Geometry: final body of the model. Coordinates: model frame, mm. A direction names the side the tool comes from. Round coordinates to 2 decimals unless told otherwise and drop trailing zeros. Loops run counter-clockwise (first coordinate to the right, second up) from the corner with the lowest first, then second, coordinate; pieces in that order, holes last. Notation, with made-up numbers: (84, 27.25) -> (110, 27.25) arc R10 cw to (110, 31.25) -> close; hole circle Ø2 at (12, 64). An arc over 180 degrees is marked (long way). Answer in a Markdown table with one row per item.
Autodesk Fusion 360 part; units mm, degrees
sketch "Sketch1" plane through (0, 0, 0) normal (0, 0, 1) x (1, 0, 0)
  line L0 (14.71, 7.35) -> (-14.71, 7.35)
  line L1 (-14.71, 7.35) -> (-14.71, -7.35)
  line L2 (-14.71, -7.35) -> (14.71, -7.35)
  line L3 (14.71, -7.35) -> (14.71, 7.35)
  line L4 (14.71, 7.35) -> (-14.71, -7.35) construction
  line L5 (-14.71, 7.35) -> (14.71, -7.35) construction
  line L6 (-17.7, 7.35) -> (-17.7, 14.7)
  line L7 (-17.7, 14.7) -> (-14.71, 14.7)
  line L8 (-17.7, 14.7) -> (17.7, 14.7)
  line L9 (17.7, 14.7) -> (17.7, -18.8)
  line L10 (17.7, -18.8) -> (-17.7, -18.8)
  line L11 (-17.7, -18.8) -> (-17.7, 14.7)
  line L12 (-17.7, 14.7) -> (6.5694, 14.7)
  line L13 (6.5694, 9.45) -> (-14.71, 9.45)
  line L14 (-17.7, 9.45) -> (-17.7, 14.7)
  line L15 (17.7, 9.45) -> (-17.7, 9.45)
  line L16 (-17.7, 9.45) -> (-17.7, -13.55)
  line L17 (-17.7, -13.55) -> (17.7, -13.55)
  line L18 (17.7, -13.55) -> (17.7, 9.45)
  line L19 (-17.7, 14.7) -> (-15.2, 14.7)
  line L20 (-15.2, 14.7) -> (-15.2, 12.2)
  line L21 (-15.2, 12.2) -> (-17.7, 12.2)
  line L22 (-17.7, 12.2) -> (-17.7, 14.7)
  circle A0 centre (-15.2, 12.2) radius 1.5
  circle A1 centre (15.2, 12.2) radius 1.5
  circle A2 centre (-15.2, -16.3) radius 1.5
  circle A3 centre (15.2, -16.3) radius 1.5
  line L23 (-17.7, -18.8) -> (-7, -18.8)
  line L24 (-7, -18.8) -> (-7, -17.6734)
  line L25 (-7, -17.6734) -> (-17.7, -17.6734)
  line L26 (-17.7, -17.6734) -> (-17.7, -18.8)
  line L27 (-7, -18.8) -> (7, -18.8)
  line L28 (7, -18.8) -> (7, -15.8)
  line L29 (7, -15.8) -> (-7, -15.8)
  line L30 (-7, -15.8) -> (-7, -18.8)
  line L31 (-17.7, 14.7) -> (-3.81, 14.7)
  line L32 (-3.81, 14.7) -> (-3.81, 12.7)
  line L33 (-3.81, 12.7) -> (-17.7, 12.7)
  line L34 (-17.7, 12.7) -> (-17.7, 14.7)
  circle A4 centre (-3.81, 12.7) radius 1
  circle A5 centre (-3.81, 12.7) radius 1
  circle A6 centre (-3.81, 12.7) radius 1
  circle A7 centre (-1.27, 12.7) radius 1
  circle A8 centre (1.27, 12.7) radius 1
  circle A9 centre (3.81, 12.7) radius 1
  circle A10 centre (-3.81, 12.7) radius 0.5
  circle A11 centre (-1.27, 12.7) radius 0.5
  circle A12 centre (1.27, 12.7) radius 0.5
  circle A13 centre (3.81, 12.7) radius 0.5
  line L35 (-2.81, 13.7) -> (-4.81, 13.7)
  line L36 (-4.81, 13.7) -> (-4.81, 11.7)
  line L37 (-4.81, 11.7) -> (-2.81, 11.7)
  line L38 (-2.81, 11.7) -> (-2.81, 13.7)
  line L39 (-2.81, 13.7) -> (-4.81, 11.7) construction
  line L40 (-4.81, 13.7) -> (-2.81, 11.7) construction
  line L41 (-0.27, 13.7) -> (-2.27, 13.7)
  line L42 (-2.27, 13.7) -> (-2.27, 11.7)
  line L43 (-2.27, 11.7) -> (-0.27, 11.7)
  line L44 (-0.27, 11.7) -> (-0.27, 13.7)
  line L45 (-0.27, 13.7) -> (-2.27, 11.7) construction
  line L46 (-2.27, 13.7) -> (-0.27, 11.7) construction
  line L47 (2.27, 13.7) -> (0.27, 13.7)
  line L48 (0.27, 13.7) -> (0.27, 11.7)
  line L49 (0.27, 11.7) -> (2.27, 11.7)
  line L50 (2.27, 11.7) -> (2.27, 13.7)
  line L51 (2.27, 13.7) -> (0.27, 11.7) construction
  line L52 (0.27, 13.7) -> (2.27, 11.7) construction
  line L53 (4.81, 13.7) -> (2.81, 13.7)
  line L54 (2.81, 13.7) -> (2.81, 11.7)
  line L55 (2.81, 11.7) -> (4.81, 11.7)
  line L56 (4.81, 11.7) -> (4.81, 13.7)
  line L57 (4.81, 13.7) -> (2.81, 11.7) construction
  line L58 (2.81, 13.7) -> (4.81, 11.7) construction
  point P0 (-3.81, 12.7)
  point P1 (-1.27, 12.7)
  point P2 (1.27, 12.7)
  point P3 (3.81, 12.7)
  dimension "d1" = 29.42
  dimension "d2" = 14.7
  dimension "d3" = 2.99
  dimension "d5" = 35.4
  dimension "d6" = 33.5
  dimension "d7" = 5.25
  dimension "d8" = 23
  dimension "d9" = 2.5
  dimension "d10" = 2.5
  dimension "d11" = 3
  dimension "d12" = 3
  dimension "d13" = 3
  dimension "d14" = 3
  dimension "d19" = 10.7
  dimension "d20" = 14
  dimension "d21" = 3
  dimension "d24" = 13.89
  dimension "d25" = 2
  dimension "d26" = 2
  dimension "d27" = 2
  dimension "d28" = 2
  dimension "d29" = 2
  dimension "d30" = 2
  dimension "d31" = 2
  dimension "d34" = 1
  dimension "d35" = 1
  dimension "d36" = 1
  dimension "d37" = 1
  dimension "d42" = 2
  dimension "d43" = 2
  dimension "d44" = 2
  dimension "d45" = 2
  dimension "d46" = 2
  dimension "d47" = 2
  dimension "d48" = 2
  dimension "d49" = 2
extrude "Extrude1" add sketch "Sketch1" along normal blind 1.2 contours L0 L1 L2 L3 | L6 L9 L11 L13 L15 L16 L17 L18 | L6 L8 L9 L11 L12 L13 L14 L15 L21 A0 L32 L33 L35 L36 L37 L38 | L9 L10 L11 L17 A2 L25 L28 L29 L30 | L6 L11 L14 L21 L22 A0 L33 | L10 L11 A2 L23 L24 L25 L26 L30 | L6 L7 L8 L11 L12 L14 L19 L20 L22 A0 L31 L33 L34 | L10 L24 L27 L28 L29 L30 | L7 L8 L12 L20 A0 L31 L32 L33 L35 L36 | L32 L33 A4 A5 A6 A10 | A4 A5 A6 L35 L36 | L32 L33 A4 A5 A6 A10 | A4 A5 A6 L36 L37 | L32 L33 A10 | L32 L33 A10 | A4 A5 A6 L35 L38 | A4 A5 A6 L37 L38 | A7 | A7 L43 L44 | A7 L41 L44 | A7 L41 L42 | A7 L42 L43 | A8 | A8 L49 L50 | A8 L47 L50 | A8 L47 L48 | A8 L48 L49 | A9 | A9 L55 L56 | A9 L53 L56 | A9 L53 L54 | A9 L54 L55 | A11 | A12 | A13 makes body 1
extrude "Extrude2" add sketch "Sketch1" along normal blind 2.7 contours L0 L1 L2 L3 | L6 L9 L11 L13 L15 L16 L17 L18 bodies 1
extrude "Extrude3" cut sketch "Sketch1" along normal blind 1.2 contours L10 L24 L27 L28 L29 L30 bodies 1
extrude "Extrude4" add sketch "Sketch1" along normal blind 2 separate body contours L32 L33 A4 A5 A6 A10 | L32 L33 A4 A5 A6 A10 | L32 L33 A10 | L32 L33 A10 | A7 | A8 | A9 | A11 | A12 | A13 makes body 2 at (-0.2712, 12.6502, 1.3333) makes body 3 at (2.2688, 12.6502, 1.3333) makes body 4 at (-2.815, 12.7996, 1.3333) makes body 5 at (4.8088, 12.6502, 1.3333)
extrude "Extrude5" add sketch "Sketch1" along normal blind 2.7 contours L32 L33 A10 | L32 L33 A10 | A11 | A12 | A13 bodies 1 2 3 4 5
chamfer "Chamfer1" distance 0.7 distance2 0.5 4 edges at (3.3438, 12.5192, 2) (0.8038, 12.5192, 2) (-1.7362, 12.5192, 2) (-4.2762, 12.5192, 2) measured on face at (4.3075, 12.7498, 2.2333) measured on face at (1.7675, 12.7498, 2.2333) measured on face at (-0.7725, 12.7498, 2.2333) measured on face at (-3.3125, 12.7498, 2.4667) on bodies 1
extrude "Extrude6" add sketch "Sketch1" against normal blind 2 contours L32 L33 A4 A5 A6 A10 | A4 A5 A6 L35 L36 | L32 L33 A4 A5 A6 A10 | A4 A5 A6 L36 L37 | L32 L33 A10 | L32 L33 A10 | A4 A5 A6 L35 L38 | A4 A5 A6 L37 L38 | A7 | A7 L43 L44 | A7 L41 L44 | A7 L41 L42 | A7 L42 L43 | A8 | A8 L49 L50 | A8 L47 L50 | A8 L47 L48 | A8 L48 L49 | A9 | A9 L55 L56 | A9 L53 L56 | A9 L53 L54 | A9 L54 L55 | A11 | A12 | A13 bodies 1
extrude "Extrude7" add sketch "Sketch1" against normal blind 8.6 contours L32 L33 A10 | L32 L33 A10 | A11 | A12 | A13 bodies 1
fillet "Fillet1" radius 0.5 4 edges at (3.3438, 12.8808, -8.6) (0.8038, 12.8808, -8.6) (-1.7362, 12.8808, -8.6) (-4.2762, 12.8808, -8.6) on bodies 1
Item 1: Draft query along X for faces 1 (the face through (-1, 11.7, -1)), 2 (the face through (-4, 12, -2)). Return one class per face: pulls with the +X half, pulls with the -X half, needs draft (parallel to the pull), parting line crosses it, or undercut.
Answer:
| item | result |
|---|---|
| face 1 | needs draft |
| face 2 | undercut |
Item 2: Cut plane D-D (x = -9). Output: boundary loops of the cut face in (y, z), then the cut area to 3 significant figures.
Answer:
| item | result |
|---|---|
| outline | (-18.8, 0) -> (14.7, 0) -> (14.7, 1.2) -> (9.45, 1.2) -> (9.45, 2.7) -> (-13.55, 2.7) -> (-13.55, 1.2) -> (-18.8, 1.2) -> close |
| area | 74.7 mm² |
Item 3: Cut plane A-A (y = -16.3). Output: boundary loops of the cut face in (x, z).
Answer:
| item | result |
|---|---|
| outline | (-17.7, 0) -> (-16.7, 0) -> (-16.7, 1.2) -> (-17.7, 1.2) -> close; (-13.7, 0) -> (-7, 0) -> (-7, 1.2) -> (-13.7, 1.2) -> close; (7, 0) -> (13.7, 0) -> (13.7, 1.2) -> (7, 1.2) -> close; (16.7, 0) -> (17.7, 0) -> (17.7, 1.2) -> (16.7, 1.2) -> close |
Item 4: Line query: probe 1 along Y at (x, z) = (-15.2, 0.7); probe 2 along Z at (x, y) = (15.5, -8.5); probe 3 along Z at (x, y) = (-8, -15). Output: solid intervals per line, ascending. Write a range as [from, to].
Answer:
| item | result |
|---|---|
| probe 1 | y = [-18.8, -17.8], [-14.8, 10.7], [13.7, 14.7] |
| probe 2 | z = [0, 2.7] |
| probe 3 | z = [0, 1.2] |
Item 5: Cut plane C-C (x = -15.2). Output: boundary loops of the cut face in (y, z).
Answer:
| item | result |
|---|---|
| outline | (-18.8, 0) -> (-17.8, 0) -> (-17.8, 1.2) -> (-18.8, 1.2) -> close; (-14.8, 0) -> (10.7, 0) -> (10.7, 1.2) -> (9.45, 1.2) -> (9.45, 2.7) -> (-13.55, 2.7) -> (-13.55, 1.2) -> (-14.8, 1.2) -> close; (13.7, 0) -> (14.7, 0) -> (14.7, 1.2) -> (13.7, 1.2) -> close |
Item 6: Reachability of faces 3 (the face through (1.205, 13.196, -5.007)), 4 (the face through (-0.81, 13.59, 1.59)), 5 (the face through (0, -15.8, 1)), 6 (the face through (-4, 13.7, -1)) from +Z, -Z, +X, -X, +Y, -Y: full face, straight path, thin tool, end or side. Return the list, or none.
Answer:
| item | result |
|---|---|
| face 3 | -Z |
| face 4 | +Z |
| face 5 | +Z, -Z, -Y |
| face 6 | -Z, +X, -X, +Y |
Item 7: Pin query (flat end, axial travel): pin 1 Ø2.5 at (x, y) = (-15.2, -16.3) entering from -Z; pin 2 Ø10 at (x, y) = (6.5, -7.5) entering from -Z; pin 3 Ø1 at (x, z) = (-6, 1.5) entering from -Y; pin 4 Ø0.5 at (x, z) = (3, 2) entering from -Y. Return the tip coordinate at first contact, or that it passes through.
Answer:
| item | result |
|---|---|
| pin 1 | passes through |
| pin 2 | stops at z = 0 |
| pin 3 | stops at y = -15.8 |
| pin 4 | stops at y = -13.55 |
Item 8: Cut plane B-B (z = -1). Output: boundary loops of the cut face in (x, y), then the cut area to 3 significant figures.
Answer:
| item | result |
|---|---|
| outline | (-4.81, 11.7) -> (-2.81, 11.7) -> (-2.81, 13.7) -> (-4.81, 13.7) -> close; (-2.27, 11.7) -> (-0.27, 11.7) -> (-0.27, 13.7) -> (-2.27, 13.7) -> close; (0.27, 11.7) -> (2.27, 11.7) -> (2.27, 13.7) -> (0.27, 13.7) -> close; (2.81, 11.7) -> (4.81, 11.7) -> (4.81, 13.7) -> (2.81, 13.7) -> close |
| area | 16.0 mm² |
